```python
from build123d import *

# Parameters (mm, degrees)
SKETCH1_R                         = 9.525
BOSS_EXTRUDE1_DEPTH               = 15.875
A_DIAMETER_DRIVE_SHAFT_SIDE_D     = 5.9436
A_DIAMETER_DRIVE_SHAFT_SIDE_DEPTH = 12.7
A_DIAMETER_DRIVE_SHAFT_SIDE_TIP   = 1.785637588
A_DIAMETER_MOTOR_SHAFT_SIDE_D     = 5.9436
A_DIAMETER_MOTOR_SHAFT_SIDE_DEPTH = 12.7
A_DIAMETER_MOTOR_SHAFT_SIDE_TIP   = 1.785637588
F_8_32_TAPPED_HOLE1_REACH         = 28.564
F_8_32_TAPPED_HOLE1_BORE_R        = 1.7272


with BuildPart() as part:
    # Sketch1 → Boss-Extrude1 (new, symmetric)
    with BuildSketch(Plane(origin=(0, 0, 0), x_dir=(0, 0, -1), z_dir=(1, 0, 0))):
        Circle(SKETCH1_R)
    extrude(amount=BOSS_EXTRUDE1_DEPTH, both=True)

    # A Diameter Drive Shaft Side
    with Locations(Plane.ZY.offset(15.875)):
        with Locations((0, 0)):
            Hole(A_DIAMETER_DRIVE_SHAFT_SIDE_D / 2, depth=A_DIAMETER_DRIVE_SHAFT_SIDE_DEPTH)
            with Locations((0, 0, -(A_DIAMETER_DRIVE_SHAFT_SIDE_DEPTH + A_DIAMETER_DRIVE_SHAFT_SIDE_TIP / 2))):  # 118° drill point
                Cone(0, A_DIAMETER_DRIVE_SHAFT_SIDE_D / 2, A_DIAMETER_DRIVE_SHAFT_SIDE_TIP, mode=Mode.SUBTRACT)

    # A Diameter Motor Shaft Side
    with Locations(Plane(origin=(15.875, 0, 0), x_dir=(0, 0, -1), z_dir=(1, 0, 0))):
        with Locations((0, 0)):
            Hole(A_DIAMETER_MOTOR_SHAFT_SIDE_D / 2, depth=A_DIAMETER_MOTOR_SHAFT_SIDE_DEPTH)
            with Locations((0, 0, -(A_DIAMETER_MOTOR_SHAFT_SIDE_DEPTH + A_DIAMETER_MOTOR_SHAFT_SIDE_TIP / 2))):  # 118° drill point
                Cone(0, A_DIAMETER_MOTOR_SHAFT_SIDE_D / 2, A_DIAMETER_MOTOR_SHAFT_SIDE_TIP, mode=Mode.SUBTRACT)

    # #8-32 Tapped Hole1 bore → #8-32 Tapped Hole1 (cut, up to next)
    with BuildSketch(Plane(origin=(0, 9.525, 0), x_dir=(1, 0, 0), z_dir=(0, 1, 0)), mode=Mode.PRIVATE) as f_8_32_tapped_hole1_sk1:
        with Locations((-8.255, 0)):
            Circle(F_8_32_TAPPED_HOLE1_BORE_R)
    f_8_32_tapped_hole1_tool1 = extrude(f_8_32_tapped_hole1_sk1.sketch, amount=-F_8_32_TAPPED_HOLE1_REACH, mode=Mode.PRIVATE) & part.part
    # #8-32 Tapped Hole1 bore → #8-32 Tapped Hole1 (cut, up to next)
    with BuildSketch(Plane(origin=(0, 9.525, 0), x_dir=(1, 0, 0), z_dir=(0, 1, 0)), mode=Mode.PRIVATE) as f_8_32_tapped_hole1_sk2:
        with Locations((8.255, 0)):
            Circle(F_8_32_TAPPED_HOLE1_BORE_R)
    f_8_32_tapped_hole1_tool2 = extrude(f_8_32_tapped_hole1_sk2.sketch, amount=-F_8_32_TAPPED_HOLE1_REACH, mode=Mode.PRIVATE) & part.part
    add(f_8_32_tapped_hole1_tool1.solids().sort_by_distance((-8.255, 9.525, 0))[0], mode=Mode.SUBTRACT)
    add(f_8_32_tapped_hole1_tool2.solids().sort_by_distance((8.255, 9.525, 0))[0], mode=Mode.SUBTRACT)


solid = part.part
```
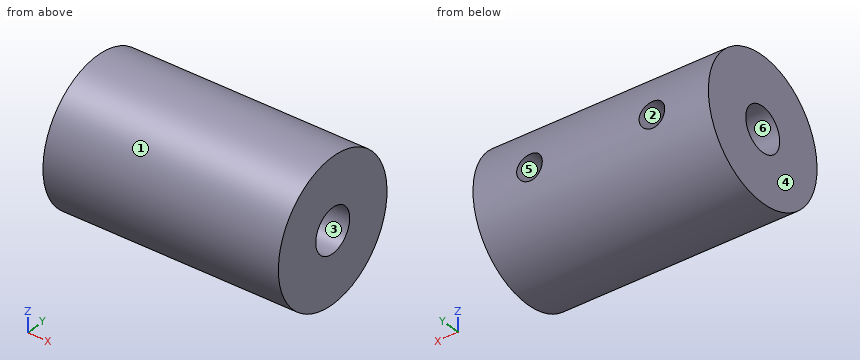
For this review, take the finished solid that the model builds, in its own axes (mm). Face numbers are marked on the shaded views. A direction names the side the tool comes from. Coordinates: 2 decimals unless noted, no trailing zeros. Order: outer loops, then holes, each group sorted by start corner. A loop starts at its lowest first (then second) coordinate and runs counter-clockwise, first axis right, second up. Notation, with made-up numbers: (9.25, 88.25) -> (17.25, 88.25) arc R11 cw to (17.25, 93.25) -> close; hole circle Ø5 at (13.25, -13.75). An arc over 180 degrees is marked (long way). Answer as CSV lines item,"result".
Q1. We need section C-C (z = 0.5). Count the separate pieces of the cut face and the enclosed holes in it, plus the area to 3 significant figures.
Model answer:
separate pieces,"3"
enclosed holes,"0"
area,"402 mm2"
Q2. Draft analysis for pull direction Y (two halves, no side actions). For the marked faces 1, 2 and 3, state which applies: released by +Y, released by -Y, zero draft, split by the parting line, or undercut.
Model answer:
face 1,"split by the parting line"
face 2,"zero draft"
face 3,"undercut"
Q3. We need section A-A (x = 12). State the section outline as (y, z) points (3 decimals), plus the area to 3 significant figures.
Model answer:
outline,"circle Ø19.05 at (0, 0); hole circle Ø5.944 at (0, 0)"
area,"257 mm2"
Q4. For the marked faces 4, 5 and 6, list the 3-axis set-ups (+Z, -Z, +X, -X, +Y, -Y) from which the entire face can be reached by the end or side of a thin tool; tool diameter is ignored.
Model answer:
face 4,"+Z, -Z, -X, +Y, -Y"
face 5,"+Y"
face 6,"-X"
Q5. We need section B-B (y = 5.5). State the section outline as (x, z) points (3 decimals), plus the area to 3 significant figures.
Model answer:
outline,"(-15.875, -7.777) -> (15.875, -7.777) -> (15.875, 7.777) -> (-15.875, 7.777) -> close; hole circle Ø3.454 at (-8.255, 0); hole circle Ø3.454 at (8.255, 0)"
area,"475 mm2"
Q6. Wall thickness on line 1 along X through (y, z) = (5.25, 0) (3 decimals); line 2 along Y through (x, z) = (14, -2); line 3 along Z through (x, y) = (1.5, 6.75): over which ranges is each line inside the solid? List them lowest first. Write a range as [from, to].
Model answer:
line 1,"x = [-15.875, -9.982], [-6.528, 6.528], [9.982, 15.875]"
line 2,"y = [-9.31, -2.2], [2.2, 9.31]"
line 3,"z = [-6.72, 6.72]"
Q7. We need section D-D (z = 8.25). State the section outline as (x, y) points (3 decimals), plus the area to 3 significant figures.
Model answer:
outline,"(-15.875, -4.761) -> (15.875, -4.761) -> (15.875, 4.761) -> (-15.875, 4.761) -> close"
area,"302 mm2"
Q8. Clearance check with flat-ended pins moving along their axes: pin 1 Ø5 at (x, y) = (-10.5, 3) entering from +Z; pin 2 Ø1 at (x, z) = (10, -3.5) entering from -Y; pin 3 Ø2 at (x, y) = (11, -3.5) entering from +Z. State where each tip first meets the part, or that it passes through.
Model answer:
pin 1,"stops at z = 9.51"
pin 2,"stops at y = -9.04"
pin 3,"stops at z = 9.19"
